Source: CAD feature listing. Evaluate the final solid. Frame: model axes, mm. Round coordinates to 2 decimals unless told otherwise and drop trailing zeros. Write each loop counter-clockwise with the first axis right and the second up, starting at its lowest first coordinate (ties: lowest second). Pieces come first, ordered by that corner, then holes.
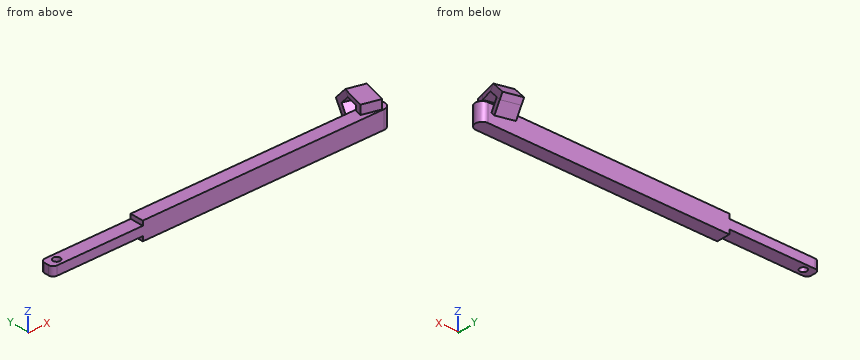
```python
from build123d import *

# Parameters (mm, degrees)
SKETCH1_R            = 2
BOSS_EXTRUDE1_DEPTH  = 10
BOSS_EXTRUDE2_DEPTH  = 5
SKETCH11_W           = 10
SKETCH11_H           = 2.5
BOSS_EXTRUDE9_DEPTH  = 10
CHAMFER4_SIZE        = 2.5
BOSS_EXTRUDE10_DEPTH = 12
BOSS_EXTRUDE11_DEPTH = 7
SKETCH14_W           = 37.56586606
SKETCH14_H           = 7.5
CUT_EXTRUDE2_DEPTH   = 99.023663822
SKETCH15_W           = 5
SKETCH15_H           = 7.5
BOSS_EXTRUDE12_DEPTH = 50
FILLET1_R            = 2.5
FILLET2_R            = 2.5
SKETCH16_R           = 2
CUT_EXTRUDE3_DEPTH   = 50


with BuildPart() as part:
    # Sketch1 → Boss-Extrude1 (new body)
    with BuildSketch(Plane.XY):
        with BuildLine():
            Line((-90, 3.75), (90, 3.75))
            ThreePointArc((90, 3.75), (93.75, 0), (90, -3.75))
            Line((90, -3.75), (-90, -3.75))
            ThreePointArc((-90, -3.75), (-93.75, 0), (-90, 3.75))
        make_face()
        with Locations((-90, 0)):
            Circle(SKETCH1_R, mode=Mode.SUBTRACT)
    extrude(amount=BOSS_EXTRUDE1_DEPTH)

    # Sketch2 → Boss-Extrude2 (add)
    with BuildSketch(Plane.XY.offset(10)):
        Polygon((80.687913142, 3.098319394), (90.347171405, 0.510128943), (89.311895225, -3.353574362), (79.652636962, -0.765383911), align=None)
    extrude(amount=BOSS_EXTRUDE2_DEPTH)

    # Sketch11 → Boss-Extrude9 (add)
    with BuildSketch(Plane(origin=(6.17964514, 23.062749635, 0), x_dir=(0.9659258262890681, -0.25881904510252146, 0), z_dir=(0.25881904510252146, 0.9659258262890681, 0))):
        with Locations((82.136635107, -13.75)):
            Rectangle(SKETCH11_W, SKETCH11_H)
    extrude(amount=BOSS_EXTRUDE9_DEPTH)

    # Chamfer4
    chamfer4_edges = [part.edges().sort_by_distance(p)[0] for p in [
        (88.105732725, 11.463482432, 12.5),
    ]]
    chamfer(chamfer4_edges, length=CHAMFER4_SIZE - 0.0001)  # a hair under: the kernel refuses the full size

    # Sketch12 → Boss-Extrude10 (add)
    with BuildSketch(Plane(origin=(2.442774957, 9.116560252, -9.438157676), x_dir=(-0.9831105418930532, 0.12706287081893997, -0.1317144231965381), z_dir=(0.18301270189222077, 0.683012701892222, -0.7071067811865448))):
        Polygon((-91.390726655, 14.25109763), (-81.565745121, 16.113820866), (-82.224317237, 19.5874764), (-92.049298771, 17.724753164), align=None)
    extrude(amount=BOSS_EXTRUDE10_DEPTH)

    # Sketch13 → Boss-Extrude11 (add)
    with BuildSketch(Plane(origin=(5.678013021, 21.19063308, 21.938157676), x_dir=(-0.9831105418930535, 0.1270628708189395, 0.13171442319653667), z_dir=(-0.18301270189221938, -0.6830127018922167, -0.70710678118655))):
        Polygon((-90.333133958, 8.672797801), (-80.508152424, 10.535521038), (-79.792866702, 6.762728129), (-89.617848236, 4.900004892), align=None)
    extrude(amount=BOSS_EXTRUDE11_DEPTH)

    # Sketch14 → Cut-Extrude2 (cut, through all)
    with BuildSketch(Plane.XY.offset(10)):
        with Locations((-62.53293303, 0)):
            Rectangle(SKETCH14_W, SKETCH14_H)
    extrude(amount=-CUT_EXTRUDE2_DEPTH, mode=Mode.SUBTRACT)


with BuildPart() as body_2:
    # of the pieces the cut leaves, the one that is kept (cut_extrude2_keep)
    add(part.part.solids().sort_by_distance((79.652636962, -0.765383911, 15))[0])

    # Sketch15 → Boss-Extrude12 (add)
    with BuildSketch(Plane.ZY.offset(43.75)):
        with Locations((5, 0)):
            Rectangle(SKETCH15_W, SKETCH15_H)
    extrude(amount=BOSS_EXTRUDE12_DEPTH)

    # Fillet1
    fillet1_edges = [body_2.edges().sort_by_distance(p)[0] for p in [
        (-93.75, 3.75, 5),
    ]]
    fillet(fillet1_edges, radius=FILLET1_R)

    # Fillet2
    fillet2_edges = [body_2.edges().sort_by_distance(p)[0] for p in [
        (-93.75, -3.75, 5),
    ]]
    fillet(fillet2_edges, radius=FILLET2_R)

    # Sketch16 → Cut-Extrude3 (cut)
    with BuildSketch(Plane.XY.offset(7.5)):
        with Locations((-88.159990551, 0)):
            Circle(SKETCH16_R)
    extrude(amount=-CUT_EXTRUDE3_DEPTH, mode=Mode.SUBTRACT)


solid = body_2.part
```
Q1. Section query A-A, the plane x = -36. Output: boundary loops of the cut face in (y, z).
Q2. Pin query (flat end, axial travel): P1, Ø3, axis at x = 38, z = 11, coming from the +Y side; P2, Ø0.8, axis at y = -1, z = 8.5, coming from the -X side; P3, Ø4, axis at y = 11.5, z = 12, coming from the +X side; P4, Ø3, axis at y = 1, z = 1.5, coming from the -X side. Return the tip coordinate at first contact, or that it passes through.
Q3. Section query B-B, the plane x = -78. Output: boundary loops of the cut face in (y, z), and give its area (3 significant figures).
Q4. Line query: line 1 (Z direction, x = -68.5, y = 1.5); line 2 (Y direction, x = 14.5, z = 4); line 3 (Z direction, x = -26, y = 1.25). Output: solid intervals per line, ascending.
Filled in:
1. outline: (-3.75, 0) - (3.75, 0) - (3.75, 10) - (-3.75, 10) - close
2. P1: stops at y = 3.75
2. P2: stops at x = -43.75
2. P3: stops at x = 93.82
2. P4: stops at x = -93.75
3. outline: (-3.75, 2.5) - (3.75, 2.5) - (3.75, 7.5) - (-3.75, 7.5) - close
3. area: 37.5 mm2
4. line 1: z = 2.5 to 7.5
4. line 2: y = -3.75 to 3.75
4. line 3: z = 0 to 10
